Autodesk Inventor part; units mm, degrees
ref_plane "YZ Plane" through (0, 0, 0) normal (1, 0, 0) x (0, 1, 0)
ref_plane "XZ Plane" through (0, 0, 0) normal (0, 1, 0) x (-1, 0, 0)
ref_plane "XY Plane" through (0, 0, 0) normal (0, 0, 1) x (1, 0, 0)
sketch "Sketch1" plane through (0, 0, 0) normal (0, 0, 1) x (1, 0, 0)
  circle A0 centre (0, 0) radius 2
  circle A1 centre (0, 0) radius 3.5
  line L0 (2, 2.8723) -> (2, -2.8723)
  line L1 (2, -2) -> (-2, -2)
  line L2 (-2, -2.8723) -> (-2, 2.8723)
  line L3 (-2.8723, 2) -> (2.8723, 2)
  dimension "d0" = 4
  dimension "d1" = 7
extrude "Extrusion1" add sketch "Sketch1" along normal blind 5 contours L0 L3 A1 | L0 A1 L3 | L2 A1 L3 | L3 A1 L2
extrude "Extrusion2" add sketch "Sketch1" against normal blind 7 contours L0 L1 A0 | L0 L3 A1 | A0 L3 L0 | A0 L2 L3 | L3 L2 A1 L0 | L1 L2 A0 | L1 L0 A1 L2 | L0 A1 L3 | L2 A1 L3 | L3 A1 L2
Input: part model. Units: mm. Frame: model coordinates. A direction names the side the tool comes from. Round coordinates to 2 decimals unless told otherwise and drop trailing zeros. Order: outer loops, then holes, each group sorted by start corner. A loop starts at its lowest first (then second) coordinate and runs counter-clockwise, first axis right, second up. Notation, with made-up numbers: (25.25, 41.5) - (82.25, 41.5) arc R33 cw to (82.25, 76.5) - close; hole circle Ø8 at (82, 83). An arc over 180 degrees is marked (long way). Answer in a Markdown table with one row per item.
Item 1: Section query C-C (z = 1.25). Return the cut outline in (x, y).
Model answer:
| item | result |
|---|---|
| outline | (-2, -2.87) - (-2, 2.87) arc R3.5 ccw to start; (2, -2.87) arc R3.5 ccw to (2, 2.87) - close |
Item 2: Reachability of faces 1 (the flat face through (-3, 0, 5)), 2 (the flat face through (2, 0, 2)) from +Z, -Z, +X, -X, +Y, -Y: full face, straight path, thin tool, end or side. Return the list, or none.
Model answer:
| item | result |
|---|---|
| face 1 | +Z, +X, -X, +Y, -Y |
| face 2 | +Z, +Y, -Y |
Item 3: Section query D-D (y = 1.75). Return the cut outline in (x, z).
Model answer:
| item | result |
|---|---|
| outline | (-3.03, -7) - (-0.97, -7) - (-0.97, 0) - (-2, 0) - (-2, 5) - (-3.03, 5) - close; (0.97, -7) - (3.03, -7) - (3.03, 5) - (2, 5) - (2, 0) - (0.97, 0) - close |
Item 4: Section query B-B (y = -1.5). Return the cut outline in (x, z).
Model answer:
| item | result |
|---|---|
| outline | (-3.16, -7) - (-1.32, -7) - (-1.32, 0) - (-2, 0) - (-2, 5) - (-3.16, 5) - close; (1.32, -7) - (3.16, -7) - (3.16, 5) - (2, 5) - (2, 0) - (1.32, 0) - close |
Item 5: Mould query, pull axis X, two halves, no side actions, for faces 3 (the flat face through (3, 0, 5)), 4 (the flat face through (-2, 0, 2)). Classes: released by +X, released by -X, zero draft, split by the parting line, or undercut.
Model answer:
| item | result |
|---|---|
| face 3 | zero draft |
| face 4 | undercut |
Item 6: Pin query (flat end, axial travel): pin 1 (4 mm diameter, centred on x = 1.5, y = -0.5, fed in from +Z); pin 2 (1.5 mm diameter, centred on x = 2.5, z = -1, fed in from -Y). Return the tip coordinate at first contact, or that it passes through.
Model answer:
| item | result |
|---|---|
| pin 1 | stops at z = 5 |
| pin 2 | stops at y = -3.03 |
Item 7: Section query A-A (x = -1.25). Return the cut outline in (y, z), then the cut area to 3 significant figures.
Model answer:
| item | result |
|---|---|
| outline | (-3.27, -7) - (-1.56, -7) - (-1.56, 0) - (-3.27, 0) - close; (1.56, -7) - (3.27, -7) - (3.27, 0) - (1.56, 0) - close |
| area | 23.9 mm² |
Item 8: Line query: line 1 (X direction, y = 0, z = -0.5); line 2 (X direction, y = -0.5, z = -2.25); line 3 (Y direction, x = 1, z = -1.25). Output: solid intervals per line, ascending.
Model answer:
| item | result |
|---|---|
| line 1 | x = -3.5 to -2, 2 to 3.5 |
| line 2 | x = -3.46 to -1.94, 1.94 to 3.46 |
| line 3 | y = -3.35 to -1.73, 1.73 to 3.35 |
